Can you work these out from the model? Positions are in its coordinate system, mm. A direction names the side the tool comes from. Give positions to 0.01 mm unless a question says otherwise; leave off trailing zeros. Loops run counter-clockwise (first coordinate to the right, second up) from the corner with the lowest first, then second, coordinate; pieces in that order, holes last. Notation, with made-up numbers: (10, 80.25) - (29, 80.25) arc R25 cw to (29, 102.25) - close; hole circle Ø4 at (19, -17). An arc over 180 degrees is marked (long way). Answer in a Markdown table with one row per item.
from build123d import *

# Parameters (mm, degrees)
SKETCH7_W           = 4.7625
SKETCH7_H           = 2.12122512
BOSS_EXTRUDE2_DEPTH = 130.175
BOSS_EXTRUDE3_DEPTH = 130.175
BOSS_EXTRUDE4_DEPTH = 130.175


with BuildPart() as part:
    # Sketch7 → Boss-Extrude2 (new, symmetric)
    with BuildSketch(Plane.XY):
        with Locations((-4.92125, -2.560612608)):
            Rectangle(SKETCH7_W, SKETCH7_H)
    extrude(amount=BOSS_EXTRUDE2_DEPTH, both=True)



with BuildPart() as body_2:
    # Sketch8 → Boss-Extrude3 (new, symmetric)
    with BuildSketch(Plane.XY):
        Polygon((2.569038147, 1.449704502), (4.950288147, 5.574150487), (6.787322988, 4.513537927), (4.406072988, 0.389091942), align=None)
    extrude(amount=BOSS_EXTRUDE3_DEPTH, both=True)


with BuildPart() as part_1:
    add(part.part)

    add(body_2.part)  # Boss-Extrude4 merges body 2
    # Sketch11 → Boss-Extrude4 (add, symmetric)
    with BuildSketch(Plane.XY):
        with BuildLine():
            Line((-2.54, -1.500000048), (-7.3025, -1.500000048))
            Line((-7.3025, -1.500000048), (-7.3025, -3.621225168))
            Line((-7.3025, -3.621225168), (-2.54, -3.621225168))
            ThreePointArc((-2.54, -3.621225168), (1.47031711, -2.546663937), (4.406072988, 0.389091942))
            Line((4.406072988, 0.389091942), (6.787322988, 4.513537927))
            Line((6.787322988, 4.513537927), (4.950288147, 5.574150487))
            Line((4.950288147, 5.574150487), (2.569038147, 1.449704502))
            Line((2.569038147, 1.449704502), (-0.029038147, 2.94970455))
            ThreePointArc((-0.029038147, 2.94970455), (-1.090295498, 1.888447198), (-2.54, 1.500000048))
            Line((-2.54, 1.500000048), (-2.54, -1.500000048))
        make_face()
    extrude(amount=BOSS_EXTRUDE4_DEPTH, both=True)


solid = part_1.part
Q1. For pin 1 (3 mm diameter, centred on x = 1.5, z = 52, fed in from +Y); pin 2 (4 mm diameter, centred on x = -2.5, z = -65, fed in from +Y); pin 3 (1.4 mm diameter, centred on x = -4.5, z = -18, fed in from +Y), each with a flat end and sliding along its axis, tell me the tip position at first contact or that it passes through.
Checked values:
| item | result |
|---|---|
| pin 1 | stops at y = 2.93 |
| pin 2 | stops at y = 2.34 |
| pin 3 | stops at y = -1.5 |
Q2. If we mould it in two halves opening along X, with no side actions, what happens to faces 1 (the face through (3.74, 3.48, 1.82)), 2 (the face through (5.613, 2.48, 1.822)), 3 (the face through (0, 0, 130.175))? For each: released by +X, released by -X, zero draft, split by the parting line, or undercut.
Checked values:
| item | result |
|---|---|
| face 1 | undercut |
| face 2 | released by +X |
| face 3 | zero draft |
Q3. If I drill on line 1 (Y direction, x = -3.75, z = 117); line 2 (X direction, y = -2.5, z = -72); line 3 (Y direction, x = 5, z = -110), over which ranges is the centre line in solid material (lowest first)? Write a range as [from, to].
Checked values:
| item | result |
|---|---|
| line 1 | y = [-3.62, -1.5] |
| line 2 | x = [-7.3, 1.55] |
| line 3 | y = [1.42, 5.55] |
Q4. Imagine slicing it at A-A, the plane z = -2. Write out the boundary of the cut face in (x, y).
Checked values:
| item | result |
|---|---|
| outline | (-7.3, -3.62) - (-2.54, -3.62) arc R8.02 ccw to (4.41, 0.39) - (6.79, 4.51) - (4.95, 5.57) - (2.57, 1.45) - (-0.03, 2.95) arc R2.9 cw to (-2.54, 1.5) - (-2.54, -1.5) - (-7.3, -1.5) - close |
Q5. On a 3-axis mill with a long thin cutter (end or side, diameter ignored), from which of +Z, -Z, +X, -X, +Y, -Y can I reach the whole of each face in a straight line? I mean faces 4 (the face through (-5, -3.621, 2)), 5 (the face through (-5, -1.5, 2)). Say none if no direction works.
Checked values:
| item | result |
|---|---|
| face 4 | +Z, -Z, +X, -X, -Y |
| face 5 | +Z, -Z, -X, +Y |
